Geometry check sheet. Reference: the model listing, model coordinates, mm. Face numbers are marked on the shaded views. A direction names the side the tool comes from. Round coordinates to 2 decimals unless told otherwise and drop trailing zeros. Order: outer loops, then holes, each group sorted by start corner. A loop starts at its lowest first (then second) coordinate and runs counter-clockwise, first axis right, second up.
(1) Cross-section at A-A on z = 18. Enter the section's corners in (x, y), and give its area (3 significant figures).
(2) Cross-section at D-D on y = -25. Enter the section's corners in (x, z), and give its area (3 significant figures).
(3) Cross-section at C-C on y = -4. Enter the section's corners in (x, z).
(4) Set-up check for the marked faces 5, 6 and 7: record each of +Z, -Z, +X, -X, +Y, -Y from which the full face is reachable in a straight line by a thin tool's end or side.
(5) Gauge pin test, flat ends, axial feed: P1, Ø8, axis at x = 7.5, y = -22.5, coming from the -Z side; P2, Ø11, axis at y = 39.72, z = 18, coming from the +X side; P3, Ø0.8, axis at x = 3, z = 9, coming from the +Y side; P4, Ø3, axis at x = 8, z = 10, coming from the -Y side. Record the tip position at first contact, or that the pin passes through.
(6) Cross-section at B-B on x = 31. Enter the section's corners in (y, z).
(7) Thickness scan on L1, parallel to Y at x = 42, z = 18; L2, parallel to Y at x = 17, z = 14.5; L3, parallel to Y at x = 52.5, z = 7.5. Record the ranges inside material, lowest first.
(8) Draft check along Z on the marked faces 1, 2, 3 and 4. Enter one of: pulls with the +Z half, pulls with the -Z half, needs draft (parallel to the pull), parting line crosses it, or undercut.
from build123d import *

# Parameters (mm, degrees)
SKETCH1_W           = 80
SKETCH1_H           = 100
BOSS_EXTRUDE1_DEPTH = 3
BOSS_EXTRUDE3_DEPTH = 80
FILLET1_R           = 5
FILLET2_R           = 5


with BuildPart() as part:
    # Sketch1 → Boss-Extrude1 (new body)
    with BuildSketch(Plane.XY):
        with Locations((18.436653688, 8.767310739)):
            Rectangle(SKETCH1_W, SKETCH1_H)
    extrude(amount=BOSS_EXTRUDE1_DEPTH)

    # Sketch3 → Boss-Extrude3 (add)
    with BuildSketch(Plane(origin=(58.436653688, 0, 0), x_dir=(0, 0, -1), z_dir=(1, 0, 0))):
        with BuildLine():
            Line((-1.837245717, 45.99131425), (-12.257916981, 45.99131425))
            ThreePointArc((-12.257916981, 45.99131425), (-16.452700501, 48.082041529), (-21.117934797, 47.631554803))
            Line((-21.117934797, 47.631554803), (-21.117934797, 45.99131425))
            ThreePointArc((-21.117934797, 45.99131425), (-11, 39.72405946), (-21.117934797, 33.45680467))
            Line((-21.117934797, 33.45680467), (-21.117934797, 31.816564117))
            ThreePointArc((-21.117934797, 31.816564117), (-16.452700501, 31.366077392), (-12.257916981, 33.45680467))
            Line((-12.257916981, 33.45680467), (-1.837245717, 33.45680467))
            Line((-1.837245717, 33.45680467), (-1.837245717, 45.99131425))
        make_face()
        with BuildLine():
            Line((-21.117934797, -13.401976374), (-21.117934797, -15.042216928))
            ThreePointArc((-21.117934797, -15.042216928), (-11, -21.309471718), (-21.117934797, -27.576726507))
            Line((-21.117934797, -27.576726507), (-21.117934797, -29.216967061))
            ThreePointArc((-21.117934797, -29.216967061), (-16.452700501, -29.667453786), (-12.257916981, -27.576726507))
            Line((-12.257916981, -27.576726507), (-1.837245717, -27.576726507))
            Line((-1.837245717, -27.576726507), (-1.837245717, -15.042216928))
            Line((-1.837245717, -15.042216928), (-11.936738174, -15.352387193))
            ThreePointArc((-11.936738174, -15.352387193), (-16.233714798, -12.995012229), (-21.117934797, -13.401976374))
        make_face()
    extrude(amount=-BOSS_EXTRUDE3_DEPTH)

    # Fillet1
    fillet1_edges = [part.edges().sort_by_distance(p)[0] for p in [
        (18.436653688, 45.99131425, 12.257916981),
        (18.436653688, 33.45680467, 12.257916981),
        (18.436653688, -15.352387193, 11.936738174),
        (18.436653688, -27.576726507, 12.257916981),
    ]]
    fillet(fillet1_edges, radius=FILLET1_R)

    # Fillet2
    fillet2_edges = [part.edges().sort_by_distance(p)[0] for p in [
        (18.436653688, 33.45680467, 3),
        (18.436653688, 45.99131425, 3),
        (18.436653688, -27.576726507, 3),
        (18.436653688, -15.077926822, 3),
    ]]
    fillet(fillet2_edges, radius=FILLET2_R)


solid = part.part
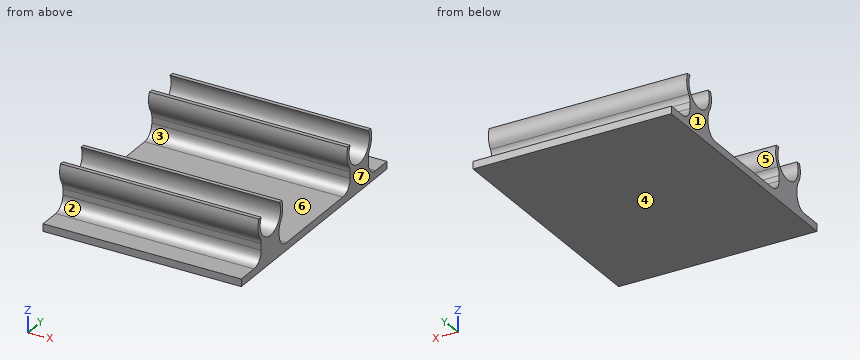
Found:
1. outline: (-21.56, -29.81) - (58.44, -29.81) - (58.44, -28.31) - (-21.56, -28.31) - close; (-21.56, -14.31) - (58.44, -14.31) - (58.44, -12.81) - (-21.56, -12.81) - close; (-21.56, 31.22) - (58.44, 31.22) - (58.44, 32.72) - (-21.56, 32.72) - close; (-21.56, 46.72) - (58.44, 46.72) - (58.44, 48.22) - (-21.56, 48.22) - close
1. area: 480 mm2
2. outline: (-21.56, 0) - (58.44, 0) - (58.44, 12.05) - (-21.56, 12.05) - close
2. area: 964 mm2
3. outline: (-21.56, 0) - (58.44, 0) - (58.44, 3) - (-21.56, 3) - close
4. face 5: +X, -X
4. face 6: +Z, +X, -X
4. face 7: +Z, -Z, +X, +Y, -Y
5. P1: stops at z = 0
5. P2: passes through
5. P3: stops at y = 45.99
5. P4: stops at y = -27.67
6. outline: (-41.23, 0) - (58.77, 0) - (58.77, 3) - (50.99, 3) arc R5 cw to (45.99, 8) - (45.99, 10.56) arc R5 cw to (46.82, 13.32) arc R8.5 ccw to (47.63, 21.12) - (45.99, 21.12) arc R7 cw (long way) to (33.46, 21.12) - (31.82, 21.12) arc R8.5 ccw to (32.63, 13.32) arc R5 cw to (33.46, 10.56) - (33.46, 8) arc R5 cw to (28.46, 3) - (-10.23, 3) arc R5 cw to (-15.23, 7.85) - (-15.29, 10.04) arc R5 cw to (-14.38, 13.08) arc R8.5 ccw to (-13.4, 21.12) - (-15.04, 21.12) arc R7 cw (long way) to (-27.58, 21.12) - (-29.22, 21.12) arc R8.5 ccw to (-28.4, 13.32) arc R5 cw to (-27.58, 10.56) - (-27.58, 8) arc R5 cw to (-32.58, 3) - (-41.23, 3) - close
7. L1: y = -29.81 to -28.31, -14.31 to -12.81, 31.22 to 32.72, 46.72 to 48.22
7. L2: y = -29.06 to -27.37, -15.25 to -13.56, 31.98 to 33.66, 45.79 to 47.47
7. L3: y = -27.6 to -15.2, 33.43 to 46.02
8. face 1: needs draft
8. face 2: undercut
8. face 3: undercut
8. face 4: pulls with the -Z half
